```python
from build123d import *

# Parameters (mm, degrees)
EXTRUDE_1_DEPTH     = 10
EXTRUDE_2_DEPTH     = 40
EXTRUDE_4_DEPTH     = 40
SKETCH_7_W          = 4
SKETCH_7_H          = 24
EXTRUDE_5_DEPTH     = 120
CUT_EXTRUDE_3_DEPTH = 95
SKETCH_10_R         = 10
EXTRUDE_6_DEPTH     = 80


with BuildPart() as part:
    # 草图1 → 凸台-拉伸1 (new body)
    with BuildSketch(Plane.XY):
        with BuildLine():
            Line((-48, 0), (-46, 0))
            ThreePointArc((-46, 0), (0, 46), (46, 0))
            Line((46, 0), (48, 0))
            ThreePointArc((48, 0), (0, 48), (-48, 0))
        make_face()
    extrude(amount=EXTRUDE_1_DEPTH)

    # 草图2 → 凸台-拉伸2 (add)
    with BuildSketch(Plane.XY.offset(10)):
        with BuildLine():
            Line((-48, 0), (-48, -12))
            Line((-48, -12), (-46, -12))
            Line((-46, -12), (-46, 0))
            ThreePointArc((-46, 0), (0, 46), (46, 0))
            Line((46, 0), (46, -12))
            Line((46, -12), (48, -12))
            Line((48, -12), (48, 0))
            ThreePointArc((48, 0), (38.88444419, 28.142494559), (15, 45.596052461))
            Line((15, 45.596052461), (15, 73))
            Line((15, 73), (10, 73))
            Line((10, 73), (10, 53))
            Line((10, 53), (-10, 53))
            Line((-10, 53), (-10, 73))
            Line((-10, 73), (-15, 73))
            Line((-15, 73), (-15, 45.596052461))
            ThreePointArc((-15, 45.596052461), (-38.88444419, 28.142494559), (-48, 0))
        make_face()
    extrude(amount=EXTRUDE_2_DEPTH)

    # 草图6 → 凸台-拉伸4 (add)
    with BuildSketch(Plane(origin=(0, 0, 10), x_dir=(-1, 0, 0), z_dir=(0, 0, -1))):
        with BuildLine():
            Line((-46, 0), (-42.166380906, 0))
            Line((-42.166380906, 0), (-42, 0))
            ThreePointArc((-42, 0), (0, 42), (42, 0))
            Line((42, 0), (46, 0))
            ThreePointArc((46, 0), (0, 46), (-46, 0))
        make_face()
    extrude(amount=-EXTRUDE_4_DEPTH)

    # 草图7 → 凸台-拉伸5 (add)
    with BuildSketch(Plane(origin=(0, 0, 10), x_dir=(-1, 0, 0), z_dir=(0, 0, -1))):
        with Locations((-44, 0)):
            Rectangle(SKETCH_7_W, SKETCH_7_H)
        with Locations((44, 0)):
            Rectangle(SKETCH_7_W, SKETCH_7_H)
    extrude(amount=-EXTRUDE_5_DEPTH)

    # 草图8 → 切除-拉伸3 (cut, through all)
    with BuildSketch(Plane.ZY.offset(46)):
        with BuildLine():
            Line((118, 12), (136, 12))
            Line((136, 12), (136, -12))
            Line((136, -12), (118, -12))
            ThreePointArc((118, -12), (130, 0), (118, 12))
        make_face()
    extrude(amount=-CUT_EXTRUDE_3_DEPTH, mode=Mode.SUBTRACT)

    # 草图10 → 凸台-拉伸6 (add, symmetric)
    with BuildSketch(Plane(origin=(0, 0, 0), x_dir=(0, 0, -1), z_dir=(1, 0, 0))):
        with Locations((-40, 59.29802623)):
            Circle(SKETCH_10_R)
    extrude(amount=EXTRUDE_6_DEPTH, both=True)


solid = part.part
```
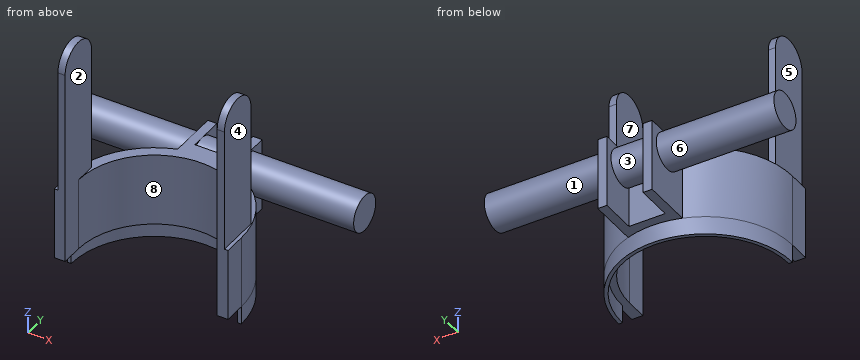
Geometry: final body of the model. Coordinates: model frame, mm. Face numbers are marked on the shaded views. A direction names the side the tool comes from. Give positions to 0.01 mm unless a question says otherwise; leave off trailing zeros. Loops run counter-clockwise (first coordinate to the right, second up) from the corner with the lowest first, then second, coordinate; pieces in that order, holes last. Notation, with made-up numbers: (-16.5, -27) -> (21.5, -27) arc R26 cw to (21.5, 1) -> close; hole circle Ø2 at (27.25, 25). An arc over 180 degrees is marked (long way). Use CSV: the item, a comma, the result in double quotes.
(1) Cut plane B-B (x = 38). Output: boundary loops of the cut face in (y, z).
From the geometry:
outline,"(17.89, 10) -> (25.92, 10) -> (25.92, 0) -> (29.33, 0) -> (29.33, 50) -> (17.89, 50) -> close; circle Ø20 at (59.3, 40)"
(2) Ray query, line 1 along X through (y, z) = (5.5, 86); line 2 along Y through (x, z) = (-45.5, 96.5); line 3 along X through (y, z) = (27.5, 20.5). Return the intervals inside material, ascending. Write a range as [from, to].
From the geometry:
line 1,"[-46, -42], [42, 46]"
line 2,"[-12, 12]"
line 3,"[-39.34, -31.75], [31.75, 39.34]"
(3) Pull-direction query (Y, two-part tool) for the marked faces 6, 7 and 8; classes: released by +Y, released by -Y, zero draft, split by the parting line, or undercut.
From the geometry:
face 6,"undercut"
face 7,"zero draft"
face 8,"released by -Y"
(4) First-contact query: P1, Ø19, axis at y = 3, z = 84, coming from the -X side; P2, Ø13, axis at y = -4, z = 23.5, coming from the -X side; P3, Ø12, axis at y = 1.5, z = 86, coming from the +X side; P4, Ø17.5, axis at x = -22, y = 20, coming from the -Z side. Flat tips, straight axial feed; report the tip coordinate or a pass-through.
From the geometry:
P1,"x = -46"
P2,"x = -48"
P3,"x = 46"
P4,"through"
(5) Cut plane C-C (z = 14). Output: boundary loops of the cut face in (x, y), plus the area to 3 significant figures.
From the geometry:
outline,"(-48, -12) -> (-42, -12) -> (-42, 0) arc R42 cw to (42, 0) -> (42, -12) -> (48, -12) -> (48, 0) arc R48 ccw to (15, 45.6) -> (15, 73) -> (10, 73) -> (10, 53) -> (-10, 53) -> (-10, 73) -> (-15, 73) -> (-15, 45.6) arc R48 ccw to (-48, 0) -> close"
area,"1,370 mm^2"
(6) Access query for the marked faces 1, 2, 3, 4 and 5. Directions: +Z, -Z, +X, -X, +Y, -Y. A direction counts if a zero-diameter tool reaches every point of the face in a straight line with its end or side. Return the directions, or none.
From the geometry:
face 1,"+X"
face 2,"+Z, -Y"
face 3,"none"
face 4,"+Z, +X, +Y, -Y"
face 5,"+Z, -X, +Y, -Y"
(7) Cut plane A-A (z = 68). Output: boundary loops of the cut face in (x, y).
From the geometry:
outline,"(-46, -12) -> (-42, -12) -> (-42, 12) -> (-46, 12) -> close; (42, -12) -> (46, -12) -> (46, 12) -> (42, 12) -> close"
(8) Cut plane D-D (y = 57). Output: boundary loops of the cut face in (x, z).
From the geometry:
outline,"(-80, 30.27) -> (-15, 30.27) -> (-15, 10) -> (-10, 10) -> (-10, 30.27) -> (10, 30.27) -> (10, 10) -> (15, 10) -> (15, 30.27) -> (80, 30.27) -> (80, 49.73) -> (15, 49.73) -> (15, 50) -> (10, 50) -> (10, 49.73) -> (-10, 49.73) -> (-10, 50) -> (-15, 50) -> (-15, 49.73) -> (-80, 49.73) -> close"
